Work out the finished part from the listing and answer in its coordinate system (mm). Face numbers are marked on the shaded views. A direction names the side the tool comes from. Coordinates: 2 decimals unless noted, no trailing zeros. Order: outer loops, then holes, each group sorted by start corner. A loop starts at its lowest first (then second) coordinate and runs counter-clockwise, first axis right, second up. Notation, with made-up numbers: (12, 6.5) -> (45, 6.5) arc R22 cw to (45, 41.5) -> close; hole circle Ø10 at (84, 59.5). An arc over 180 degrees is marked (long way). Use one line per item in the form item = value.
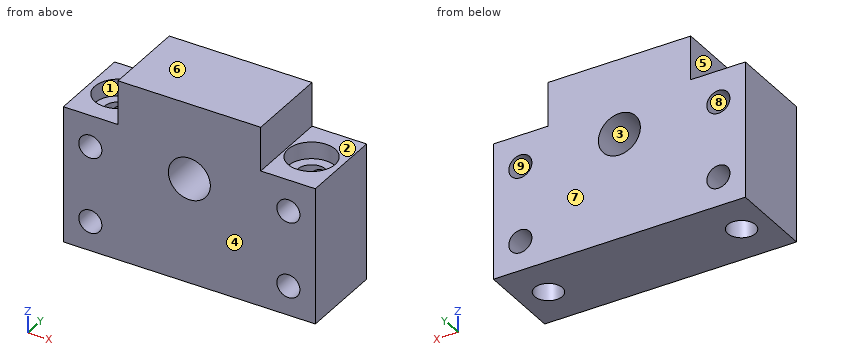
from build123d import *

# Parameters (mm, degrees)
F0_R           = 5
F1_DEPTH       = 20
F3_D           = 6.6
F3_CBORE_D     = 11.25
F3_CBORE_DEPTH = 4
F4_D           = 5.5


with BuildPart() as f1:
    # F0 (on Front) → F1 (new body)
    with BuildSketch(Plane.XZ):
        Polygon((30, -16.25), (30, 16.25), (17, 16.25), (17, 26.75), (-17, 26.75), (-17, 16.25), (-30, 16.25), (-30, -16.25), align=None)
        with Locations((0, 8.75)):
            Circle(F0_R, mode=Mode.SUBTRACT)
    extrude(amount=F1_DEPTH)

    # F3 (through all)
    with Locations(Plane.XY.offset(16.25)):
        with Locations((-23, -10), (23, -10)):
            CounterBoreHole(F3_D / 2, F3_CBORE_D / 2, F3_CBORE_DEPTH)

    # F4 (through all)
    with Locations(Plane(origin=(0, 0, 0), x_dir=(1, 0, 0), z_dir=(0, 1, 0))):
        with Locations((23.5833972692, -8.75), (23.5833972692, 9.25), (-23.5833972692, 9.25), (-23.5833972692, -8.75)):
            Hole(F4_D / 2)


solid = f1.part
(1) Straight lines are drawn through the part: line 1 along Y through (x, z) = (23, 14) (3 decimals); line 2 along X through (y, z) = (-12.5, -9.25); line 3 along Y through (x, z) = (-23, -6). For each, find the intervals that lie inside material, in ascending order.
Data:
line_1 = -20 to -15.625, -4.375 to 0
line_2 = -30 to -26.33, -20.83 to 20.83, 26.33 to 30
line_3 = -20 to -13.3, -6.7 to 0
(2) The mould has two halves that part along Z. Classify the marked faces 6, 7, 8 and 9: released by +Z, released by -Z, zero draft, split by the parting line, or undercut.
Data:
face_6 = released by +Z
face_7 = zero draft
face_8 = undercut
face_9 = undercut
(3) Section C-C on z = -3.5 is taken. Write down the section's boundary in (x, y), plus the area to 3 significant figures.
Data:
outline = (-30, -20) -> (30, -20) -> (30, 0) -> (-30, 0) -> close; hole circle Ø6.6 at (-23, -10); hole circle Ø6.6 at (23, -10)
area = 1,130 mm²
(4) Which of the six approach directions +Z, -Z, +X, -X, +Y, -Y give full straight-line access (tool end or side, diameter ignored) to the marked faces 1, 2, 3, 4 and 5?
Data:
face_1 = +Z
face_2 = +Z, +X, +Y, -Y
face_3 = +Y, -Y
face_4 = +Z, -Z, +X, -X, -Y
face_5 = +Z, -X, +Y, -Y
(5) Each of these flat-tipped pins is pushed along its axis until it touches: P1, Ø3.5, axis at x = -23.5, y = -7.5, coming from the +Z side; P2, Ø11.5, axis at y = -6, z = 23, coming from the +X side; P3, Ø6.5, axis at x = -21, y = -7.5, coming from the +Z side. Where does it stop, or does it pass through?
Data:
P1 = 12.25
P2 = 17
P3 = 16.25
(6) Section B-B on y = -10 is taken. Count the separate pieces of the cut face and the enclosed holes in it, plus the area to 3 significant figures.
Data:
separate_pieces = 3
enclosed_holes = 1
area = 1,760 mm²
(7) Section A-A on x = 24 is taken. Write down the section's boundary in (y, z).
Data:
outline = (-20, -16.25) -> (-13.14, -16.25) -> (-13.14, -11.97) -> (-20, -11.97) -> close; (-20, -6.53) -> (-13.14, -6.53) -> (-13.14, 6.03) -> (-20, 6.03) -> close; (-20, 11.47) -> (-13.14, 11.47) -> (-13.14, 12.25) -> (-15.54, 12.25) -> (-15.54, 16.25) -> (-20, 16.25) -> close; (-6.86, -16.25) -> (0, -16.25) -> (0, -11.97) -> (-6.86, -11.97) -> close; (-6.86, -6.53) -> (0, -6.53) -> (0, 6.03) -> (-6.86, 6.03) -> close; (-6.86, 11.47) -> (0, 11.47) -> (0, 16.25) -> (-4.46, 16.25) -> (-4.46, 12.25) -> (-6.86, 12.25) -> close
(8) Section D-D on x = 4 is taken. Write down the section's boundary in (y, z).
Data:
outline = (-20, -16.25) -> (0, -16.25) -> (0, 5.75) -> (-20, 5.75) -> close; (-20, 11.75) -> (0, 11.75) -> (0, 26.75) -> (-20, 26.75) -> close
